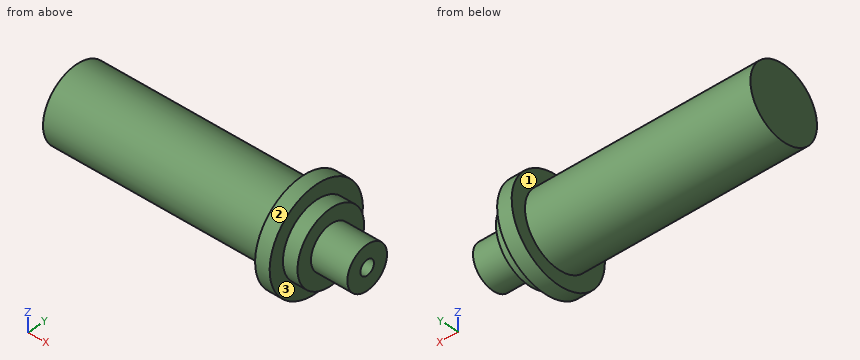
```python
from build123d import *

# Parameters (mm, degrees)
F0_W   = 2.54
F0_H   = 6.35
F0_H_2 = 2.54
F0_W_2 = 39.37
F0_W_3 = 6.35
F0_H_3 = 2.4892


# Not quite as in the source:
# - a feature names something its author has since deleted; it is built from what else it names


with BuildPart() as f1:
    # F0 (on Front) → F1 (revolve)
    with BuildSketch(Plane.XZ):
        Polygon((-23.0985377062, 28.9715196595), (-25.6385377062, 28.9715196595), (-25.6385377062, 22.6215196595), (-23.0985377062, 22.6215196595), (-23.0985377062, 23.9169196595), (-23.0985377062, 26.4061196595), align=None)
        with Locations((-26.9085377062, 25.7965196595)):
            Rectangle(F0_W, F0_H)
        with Locations((-26.9085377062, 30.2415196595)):
            Rectangle(F0_W, F0_H_2)
        with Locations((-47.8635377062, 25.7965196595)):
            Rectangle(F0_W_2, F0_H)
        with Locations((-19.9235377062, 25.1615196595)):
            Rectangle(F0_W_3, F0_H_3)
    revolve(axis=Axis((-42.1485377062, 0, 22.6215196595), (1, 0, 0)))


solid = f1.part
```
Geometry check sheet. Reference: the model listing, model coordinates, mm. Face numbers are marked on the shaded views. A direction names the side the tool comes from. Coordinates: 2 decimals unless noted, no trailing zeros. Loops run counter-clockwise (first coordinate to the right, second up) from the corner with the lowest first, then second, coordinate; pieces in that order, holes last.
Item 1: Go/stop test with flat-tipped pins: pin 1 Ø1 at (x, z) = (-43.5, 28) entering from +Y; pin 2 Ø2 at (y, z) = (0, 22.62) entering from +X; pin 3 Ø2 at (x, z) = (-54, 17.5) entering from -Y. Record where each tip stops, or that it passes through.
Item 2: Sectioned sample at A-A, the plane y = 0. Record the boundary of the cut face in (x, z), then the cut area to 3 significant figures.
Item 3: Thickness scan on line 1 (Z direction, x = -19.25, y = 0); line 2 (X direction, y = -2.25, z = 27.5); line 3 (X direction, y = -5.75, z = 19). Record the ranges inside material, lowest first.
Item 4: Sectioned sample at B-B, the plane x = -54. Record the boundary of the cut face in (y, z).
Item 5: Access from +Z, -Z, +X, -X, +Y, -Y to the whole of each face (thin tool, end or side, straight path). Record for the marked faces 1, 2 and 3.
Item 6: Sectioned sample at C-C, the plane y = 2.75. Record the boundary of the cut face in (x, z).
Item 7: Sectioned sample at D-D, the plane y = -4.75. Record the boundary of the cut face in (x, z).
Check result:
1. pin 1: stops at y = 4.06
1. pin 2: stops at x = -23.1
1. pin 3: stops at y = -4.83
2. outline: (-67.55, 16.27) - (-28.18, 16.27) - (-28.18, 13.73) - (-25.64, 13.73) - (-25.64, 16.27) - (-23.1, 16.27) - (-23.1, 18.84) - (-16.75, 18.84) - (-16.75, 21.33) - (-23.1, 21.33) - (-23.1, 23.92) - (-16.75, 23.92) - (-16.75, 26.41) - (-23.1, 26.41) - (-23.1, 28.97) - (-25.64, 28.97) - (-25.64, 31.51) - (-28.18, 31.51) - (-28.18, 28.97) - (-67.55, 28.97) - close
2. area: 609 mm2
3. line 1: z = 18.84 to 21.33, 23.92 to 26.41
3. line 2: x = -67.55 to -23.1
3. line 3: x = -28.18 to -25.64
4. outline: circle Ø12.7 at (0, 22.62)
5. face 1: -X
5. face 2: +X, -X
5. face 3: +X
6. outline: (-67.55, 16.9) - (-28.18, 16.9) - (-28.18, 14.17) - (-25.64, 14.17) - (-25.64, 16.9) - (-23.1, 16.9) - (-23.1, 20.02) - (-16.75, 20.02) - (-16.75, 25.22) - (-23.1, 25.22) - (-23.1, 28.35) - (-25.64, 28.35) - (-25.64, 31.08) - (-28.18, 31.08) - (-28.18, 28.35) - (-67.55, 28.35) - close
7. outline: (-67.55, 18.41) - (-28.18, 18.41) - (-28.18, 15.11) - (-25.64, 15.11) - (-25.64, 18.41) - (-23.1, 18.41) - (-23.1, 26.84) - (-25.64, 26.84) - (-25.64, 30.14) - (-28.18, 30.14) - (-28.18, 26.84) - (-67.55, 26.84) - close
